```python
from build123d import *

# Parameters (mm, degrees)
BOX001027045134_W           = 10
BOX001027045134_H           = 10
BOX001027045134_DEPTH       = 32
CYLINDER192_R               = 2.2
CYLINDER192_DEPTH           = 17
CUT158_PLACEMENT_ANGLE      = 180
BOX001027045133_W           = 10
BOX001027045133_H           = 10
BOX001027045133_DEPTH       = 32
BOX001027045132_W           = 15
BOX001027045132_H           = 10
BOX001027045132_DEPTH       = 18
BOX001027045135_W           = 25
BOX001027045135_H           = 10
BOX001027045135_DEPTH       = 25
TORUS013_R                  = 2.2
TORUS013_ROLL_ANGLE         = 90
COMMON091_PITCH_ANGLE       = -45
COMMON090_PLACEMENT_ANGLE   = 180
CYLINDER191_R               = 2.2
CYLINDER191_DEPTH           = 9
CYLINDER193_R               = 2.2
CYLINDER193_DEPTH           = 9
CYLINDER190_R               = 1.15
CYLINDER190_DEPTH           = 32
CYLINDER171_R               = 1.75
CYLINDER171_DEPTH           = 30
CYLINDER171_ROLL_ANGLE      = 90
CYLINDER195_R               = 1.75
CYLINDER195_DEPTH           = 30
CYLINDER195_ROLL_ANGLE      = 90
BOX001027045140_W           = 26
BOX001027045140_H           = 21
BOX001027045140_DEPTH       = 6
CYLINDER189_R               = 5
CYLINDER189_DEPTH           = 8
CYLINDER189_ROLL_ANGLE      = 90
BOX001027045139_W           = 21
BOX001027045139_H           = 10
BOX001027045139_DEPTH       = 28
BOX001027045139_PITCH_ANGLE = 45
BOX001027045138_W           = 21
BOX001027045138_H           = 10
BOX001027045138_DEPTH       = 28
BOX001027045137_W           = 21
BOX001027045137_H           = 8
BOX001027045137_DEPTH       = 28


with BuildPart() as cube187:
    # Box001027045134 → Box001027045134 (new body)
    with BuildSketch(Plane(origin=(0, -5, -22), x_dir=(1, 0, 0), z_dir=(0, 0, 1))):
        with Locations((5, 5)):
            Rectangle(BOX001027045134_W, BOX001027045134_H)
    extrude(amount=BOX001027045134_DEPTH)


with BuildPart() as cut158:
    # Cylinder192 → Cylinder192 (new body)
    with BuildSketch(Plane.XY.offset(-15)):
        Circle(CYLINDER192_R)
    extrude(amount=CYLINDER192_DEPTH)

    # Cut158: cut Cube187
    add(cube187.part, mode=Mode.SUBTRACT)


with BuildPart() as cut158_1:
    # Cut158 placement: moved
    add(cut158.part.moved(Location((0, 0, 6))).rotate(Axis((0, 0, 6), (1, 0, 0)), CUT158_PLACEMENT_ANGLE))


with BuildPart() as cube186:
    # Box001027045133 → Box001027045133 (new body)
    with BuildSketch(Plane(origin=(0, -5, -22), x_dir=(1, 0, 0), z_dir=(0, 0, 1))):
        with Locations((5, 5)):
            Rectangle(BOX001027045133_W, BOX001027045133_H)
    extrude(amount=BOX001027045133_DEPTH)


with BuildPart() as cube185:
    # Box001027045132 → Box001027045132 (new body)
    with BuildSketch(Plane(origin=(-5, -5, -18), x_dir=(1, 0, 0), z_dir=(0, 0, 1))):
        with Locations((7.5, 5)):
            Rectangle(BOX001027045132_W, BOX001027045132_H)
    extrude(amount=BOX001027045132_DEPTH)


with BuildPart() as cube188:
    # Box001027045135 → Box001027045135 (new body)
    with BuildSketch(Plane(origin=(-3, -5, -1), x_dir=(1, 0, 0), z_dir=(0, 0, 1))):
        with Locations((12.5, 5)):
            Rectangle(BOX001027045135_W, BOX001027045135_H)
    extrude(amount=BOX001027045135_DEPTH)


with BuildPart() as common090:
    # Torus013 → Torus013 (revolve)
    with BuildSketch(Plane.XZ):
        with Locations((20, 0)):
            Circle(TORUS013_R)
    revolve(axis=Axis((0, 0, 0), (0, 0, 1)))


with BuildPart() as common090_1:
    # Torus013 roll: moved
    add(common090.part.rotate(Axis((0, 0, 0), (1, 0, 0)), TORUS013_ROLL_ANGLE))


with BuildPart() as common090_2:
    # Torus013 placement: moved
    add(common090_1.part.moved(Location((20, 0, 0))))

    # Common091: intersect Cube188
    add(cube188.part, mode=Mode.INTERSECT)


with BuildPart() as common090_3:
    # Common091 pitch: moved
    add(common090_2.part.rotate(Axis((0, 0, 0), (0, 1, 0)), COMMON091_PITCH_ANGLE))


with BuildPart() as common090_4:
    # Common091 placement: moved
    add(common090_3.part.moved(Location((5.857864, 0, -14.142136))))

    # Common089: intersect Cube185
    add(cube185.part, mode=Mode.INTERSECT)

    # Common090: intersect Cube186
    add(cube186.part, mode=Mode.INTERSECT)


with BuildPart() as common090_5:
    # Common090 placement: moved
    add(common090_4.part.moved(Location((0, 0, 4))).rotate(Axis((0, 0, 4), (1, 0, 0)), COMMON090_PLACEMENT_ANGLE))


with BuildPart() as cylinder238:
    # Cylinder191 → Cylinder191 (new body)
    with BuildSketch(Plane(origin=(0, 0, 4), x_dir=(1, 0, 0), z_dir=(0, 0, -1))):
        Circle(CYLINDER191_R)
    extrude(amount=CYLINDER191_DEPTH)


with BuildPart() as cylinder240:
    # Cylinder193 → Cylinder193 (new body)
    with BuildSketch(Plane(origin=(0, 0, 33), x_dir=(1, 0, 0), z_dir=(0, 0, -1))):
        Circle(CYLINDER193_R)
    extrude(amount=CYLINDER193_DEPTH)


with BuildPart() as cylinder237:
    # Cylinder190 → Cylinder190 (new body)
    with BuildSketch(Plane(origin=(0, 0, 30), x_dir=(1, 0, 0), z_dir=(0, 0, -1))):
        Circle(CYLINDER190_R)
    extrude(amount=CYLINDER190_DEPTH)


with BuildPart() as filament_path002:
    # Fusion112095 base: copy of Cylinder237
    add(cylinder237.part)

    # Fusion112095: union Cut158, Common090, Cylinder238, Cylinder240
    add(cut158_1.part)
    add(common090_5.part)
    add(cylinder238.part)
    add(cylinder240.part)


with BuildPart() as filament_path002_1:
    # Fusion112095 placement: moved
    add(filament_path002.part.moved(Location((0, 0, 5))))


with BuildPart() as top_path:
    # Fusion112086 base: copy of Cylinder237
    add(cylinder237.part)

    # Fusion112086: union Cut158, Common090, Cylinder238, Cylinder240
    add(cut158_1.part)
    add(common090_5.part)
    add(cylinder238.part)
    add(cylinder240.part)


with BuildPart() as top_path_1:
    # Fusion112086 placement: moved
    add(top_path.part.moved(Location((0, 0, -23))))

    # Fusion112096: union filament-path002
    add(filament_path002_1.part)


with BuildPart() as m3_clear:
    # Cylinder171 → Cylinder171 (new body)
    with BuildSketch(Plane.XY):
        Circle(CYLINDER171_R)
    extrude(amount=CYLINDER171_DEPTH)


with BuildPart() as m3_clear_1:
    # Cylinder171 roll: moved
    add(m3_clear.part.rotate(Axis((0, 0, 0), (1, 0, 0)), CYLINDER171_ROLL_ANGLE))


with BuildPart() as m3_clear_2:
    # Cylinder171 placement: moved
    add(m3_clear_1.part.moved(Location((7, 13, 15))))


with BuildPart() as top_m3_clear:
    # Cylinder195 → Cylinder195 (new body)
    with BuildSketch(Plane.XY):
        Circle(CYLINDER195_R)
    extrude(amount=CYLINDER195_DEPTH)


with BuildPart() as top_m3_clear_1:
    # Cylinder195 roll: moved
    add(top_m3_clear.part.rotate(Axis((0, 0, 0), (1, 0, 0)), CYLINDER195_ROLL_ANGLE))


with BuildPart() as top_m3_clear_2:
    # Cylinder195 placement: moved
    add(top_m3_clear_1.part.moved(Location((-6, 13, -1))))

    # Fusion112093: union M3-clear
    add(m3_clear_2.part)


with BuildPart() as cube193:
    # Box001027045140 → Box001027045140 (new body)
    with BuildSketch(Plane(origin=(-6, -4, 2), x_dir=(1, 0, 0), z_dir=(0, 0, 1))):
        with Locations((13, 10.5)):
            Rectangle(BOX001027045140_W, BOX001027045140_H)
    extrude(amount=BOX001027045140_DEPTH)


with BuildPart() as screw_bump_top:
    # Cylinder189 → Cylinder189 (new body)
    with BuildSketch(Plane.XY):
        Circle(CYLINDER189_R)
    extrude(amount=CYLINDER189_DEPTH)


with BuildPart() as screw_bump_top_1:
    # Cylinder189 roll: moved
    add(screw_bump_top.part.rotate(Axis((0, 0, 0), (1, 0, 0)), CYLINDER189_ROLL_ANGLE))


with BuildPart() as screw_bump_top_2:
    # Cylinder189 placement: moved
    add(screw_bump_top_1.part.moved(Location((-6, 0, -1))))


with BuildPart() as cube192:
    # Box001027045139 → Box001027045139 (new body)
    with BuildSketch(Plane.XY):
        with Locations((10.5, 5)):
            Rectangle(BOX001027045139_W, BOX001027045139_H)
    extrude(amount=BOX001027045139_DEPTH)


with BuildPart() as cube192_1:
    # Box001027045139 pitch: moved
    add(cube192.part.rotate(Axis((0, 0, 0), (0, 1, 0)), BOX001027045139_PITCH_ANGLE))


with BuildPart() as cube192_2:
    # Box001027045139 placement: moved
    add(cube192_1.part.moved(Location((-6, -9, 21))))


with BuildPart() as fusion112087:
    # Box001027045138 → Box001027045138 (new body)
    with BuildSketch(Plane(origin=(-6, -9, -7), x_dir=(1, 0, 0), z_dir=(0, 0, 1))):
        with Locations((10.5, 5)):
            Rectangle(BOX001027045138_W, BOX001027045138_H)
    extrude(amount=BOX001027045138_DEPTH)

    # Fusion112087: union Cube192
    add(cube192_2.part)


with BuildPart() as fusion112087_1:
    # Fusion112087 placement: moved
    add(fusion112087.part.moved(Location((10, 0, -17))))


with BuildPart() as top:
    # Box001027045137 → Box001027045137 (new body)
    with BuildSketch(Plane(origin=(-6, -8, -7), x_dir=(1, 0, 0), z_dir=(0, 0, 1))):
        with Locations((10.5, 4)):
            Rectangle(BOX001027045137_W, BOX001027045137_H)
    extrude(amount=BOX001027045137_DEPTH)

    # Cut160: cut Fusion112087
    add(fusion112087_1.part, mode=Mode.SUBTRACT)

    # Fusion112088: union screw-bump-top
    add(screw_bump_top_2.part)

    # Cut161: cut Cube193
    add(cube193.part, mode=Mode.SUBTRACT)

    # Cut167: cut top-m3-clear
    add(top_m3_clear_2.part, mode=Mode.SUBTRACT)

    # Cut170: cut top-path
    add(top_path_1.part, mode=Mode.SUBTRACT)


solid = top.part
```
CAD build for the part. Positions are in the model's coordinates, mm. A direction names the side the tool comes from. Round coordinates to 2 decimals unless told otherwise and drop trailing zeros. Loops run counter-clockwise (first coordinate to the right, second up) from the corner with the lowest first, then second, coordinate; pieces in that order, holes last. Notation, with made-up numbers: M 1,64.5 L 28,64.5 A21 cw 28,81.5 Z; hole C -25.75,86 d1. An arc over 180 degrees is marked long. Return JSON: item names as keys, results as strings. Group by question number.
(1) Mould opens along Z. For faces 4 (the cylindrical face through (-1.54, -1.57, -4.46)), 5 (the flat face through (-1, -4, 5)), 6 (the flat face through (-1.1, -2.4, 2)), 7 (the flat face through (11, -4, 11)) say: +Z half, -Z half, draft (parallel to the pull), parting line (faces both ways), or undercut.
(2) Saw through at B-B, the plane y = -7. List the corners of the cut face in (x, z), and give its area (3 significant figures).
(3) Wall check: probe 1 along X at (y, z) = (-2, 14.75); probe 2 along Z at (x, y) = (13.25, -6.5); probe 3 along Z at (x, y) = (5.5, -2.25). Give the ranges that are in metal, low to high. Write a range as [from, to].
(4) Saw through at A-A, the plane z = -1. List the corners of the cut face in (x, y).
(5) Saw through at C-C, the plane x = 9.5. List the corners of the cut face in (y, z).
(6) Tool access for faces 1 (the cylindrical face through (0.497, -1.037, 20.15)), 2 (the flat face through (-6, -2, 3)), 3 (the flat face through (-1, -1, -2)): list every direction of +Z, -Z, +X, -X, +Y, -Y with a clear straight run to the whole face (end or side of a thin tool).
(7) Drop flat-ended pins along their axis: P1, Ø0.5, axis at y = -1.5, z = -4, coming from the -X side; P2, Ø0.5, axis at y = -1.5, z = 14, coming from the -X side; P3, Ø0.6, axis at y = -1.5, z = 3, coming from the +X side. Give the stop position or say it passes through.
(8) Saw through at D-D, the plane z = 6.25. List the corners of the cut face in (x, y), and give its area (3 significant figures).
Answer list:
{
 "1": {"face 4": "draft", "face 5": "undercut", "face 6": "undercut", "face 7": "-Z half"},
 "2": {"outline": "M -6,-7 L 4,-7 L 4,4 L 15,15 L 15,21 L -6,21 L -6,4 A5 ccw -6,-6 Z; hole C -6,-1 d3.5; hole C 7,15 d3.5", "area": "427 mm2"},
 "3": {"probe 1": "[-6, -0.92], [1.8, 5.27], [8.73, 14.75]", "probe 2": "[13.25, 21]", "probe 3": "[8, 14.1], [15.9, 21]"},
 "4": {"outline": "M -11,-8 L -7.75,-8 L -7.75,0 L -11,0 Z; M -4.25,-8 L 4,-8 L 4,0 L 1.15,0 A1.15 cw -1.15,0 L -4.25,0 Z"},
 "5": {"outline": "M -8,9.5 L 0,9.5 L 0,21 L -8,21 Z"},
 "6": {"face 1": "+Z, -Z, +Y", "face 2": "+X, +Y", "face 3": "-Z, +Y"},
 "7": {"P1": "x = -10.18", "P2": "x = -6", "P3": "x = -6"},
 "8": {"outline": "M -6,-8 L 6.25,-8 L 6.25,-4 L -6,-4 Z", "area": "49.0 mm2"}
}
